Job drawing, mm, ordinate dimensions from the low corner. One solid piece. A direction names the side the tool comes from. Coordinates: 2 decimals unless noted, no trailing zeros. Write each loop counter-clockwise with the first axis right and the second up, starting at its lowest first coordinate (ties: lowest second). Pieces come first, ordered by that corner, then holes.
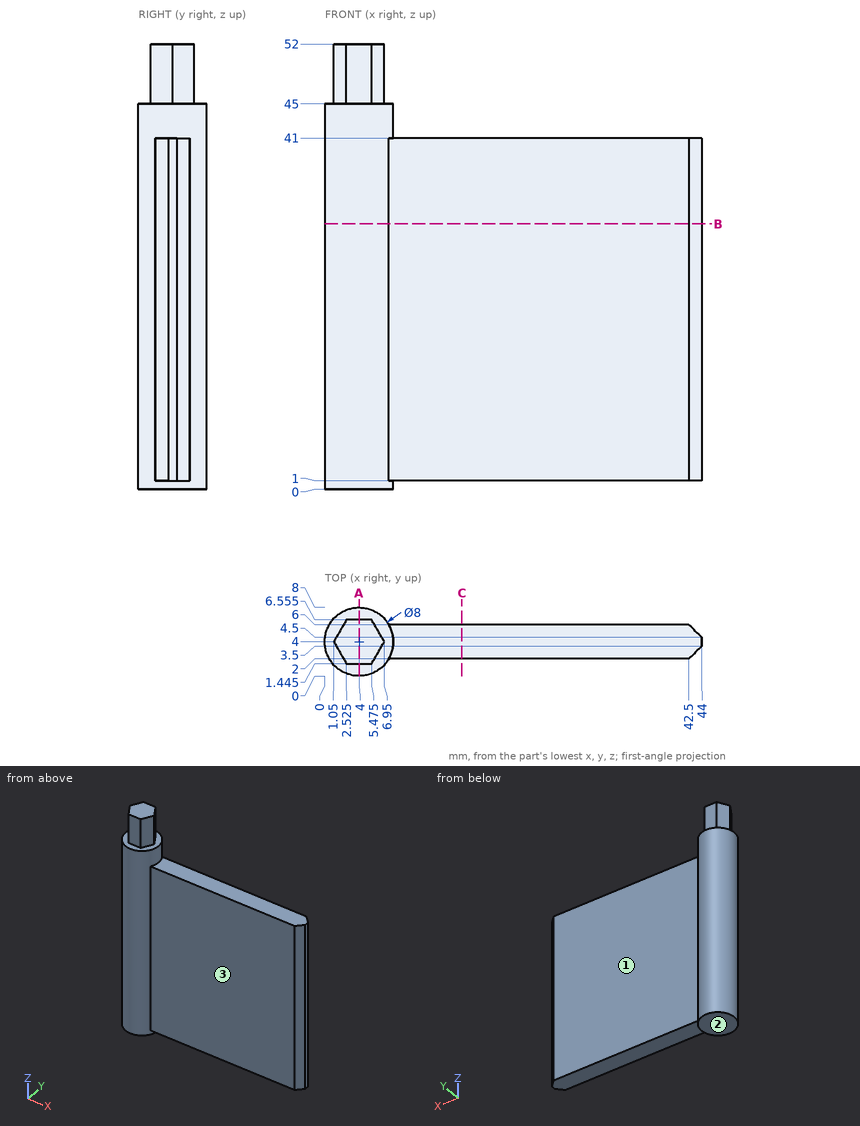
1. 3-axis set-ups, long thin cutter, end or side, ignore diameter. For the marked faces 1, 2 and 3: which of +Z, -Z, +X, -X, +Y, -Y reach the whole face in a straight line?
Computed values:
face 1: +Z, -Z, +X, +Y
face 2: -Z, +X, -X, +Y, -Y
face 3: +Z, -Z, +X, -Y
2. Saw through at B-B on z = 31. List the corners of the cut face in (x, y).
Computed values:
outline: (7.46, 2) - (42.5, 2) - (44, 3.5) - (44, 4.5) - (42.5, 6) - (7.46, 6) arc R4 ccw (long way) to start
3. Saw through at A-A on x = 4. List the corners of the cut face in (y, z) (1 decimal), plus the area to 3 significant figures.
Computed values:
outline: (0, 0) - (8, 0) - (8, 45) - (6.6, 45) - (6.6, 52) - (1.4, 52) - (1.4, 45) - (0, 45) - close
area: 396 mm2
4. Saw through at C-C on x = 16. List the corners of the cut face in (y, z), plus the area to 3 significant figures.
Computed values:
outline: (2, 1) - (6, 1) - (6, 41) - (2, 41) - close
area: 160 mm2
5. Probe line 1 along Z through (x, y) = (33.5, 4.75); line 2 along Z through (x, y) = (2, 1.25); line 3 along Y through (x, z) = (25, 36). List the from-to ranges inside material, lowest first.
Computed values:
line 1: z = 1 to 41
line 2: z = 0 to 45
line 3: y = 2 to 6
6. Flat gauge pins, fed straight in: pin 1 (3 mm diameter, centred on x = 4.5, z = 49.5, fed in from +Y) (3 decimals); pin 2 (4 mm diameter, centred on y = 7, z = 32.5, fed in from +X); pin 3 (3 mm diameter, centred on x = 22, y = 4, fed in from -Z). Where does each tip first touch, or does it go through?
Computed values:
pin 1: stops at y = 6.555
pin 2: stops at x = 43.5
pin 3: stops at z = 1
